```python
from build123d import *

# Parameters (mm, degrees)
F0_R     = 10
F1_DEPTH = 16
F2_R     = 1
F3_R     = 1


with BuildPart() as f1:
    # F0 (on Front) → F1 (new body)
    with BuildSketch(Plane.XZ):
        Polygon((-20, -11.547005), (0, -23.094011), (20, -11.547005), (20, 11.547005), (0, 23.094011), (-20, 11.547005), align=None)
        Circle(F0_R, mode=Mode.SUBTRACT)
    extrude(amount=F1_DEPTH)

    # F2
    f2_edges = [f1.edges().sort_by_distance(p)[0] for p in [
        (-20, -16, 0),
        (-10, -16, -17.320508),
        (10, -16, -17.320508),
        (20, -16, 0),
        (10, -16, 17.320508),
        (-10, -16, 17.320508),
        (-10, -16, 0),
    ]]
    fillet(f2_edges, radius=F2_R)

    # F3
    f3_edges = [f1.edges().sort_by_distance(p)[0] for p in [
        (-20, 0, 0),
        (-10, 0, -17.320508),
        (10, 0, -17.320508),
        (20, 0, 0),
        (10, 0, 17.320508),
        (-10, 0, 17.320508),
        (-10, 0, 0),
    ]]
    fillet(f3_edges, radius=F3_R)


solid = f1.part
```
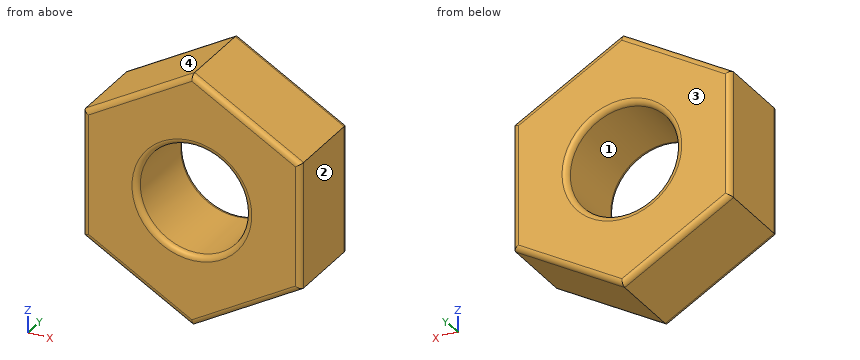
Input: part model. Units: mm. Frame: model coordinates. Face numbers are marked on the shaded views. Give positions to 0.01 mm unless a question says otherwise; leave off trailing zeros. Order: outer loops, then holes, each group sorted by start corner. A loop starts at its lowest first (then second) coordinate and runs counter-clockwise, first axis right, second up. Notation, with made-up numbers: M 50.25,86.5 L 73.25,86.5 A20 cw 73.25,96.5 Z; hole C 70,68.5 d2. An arc over 180 degrees is marked long. One line per question, with ' | ' between items.
1) Ray query, L1, parallel to Y at x = 1, z = 21.5; L2, parallel to Z at x = 3.5, y = -7.25; L3, parallel to X at y = -14.75, z = 8.5. Return the intervals inside material, ascending.
Filled in:
L1: y = -15.99 to -0.01 | L2: z = -21.07 to -9.37, 9.37 to 21.07 | L3: x = -20 to -5.27, 5.27 to 20
2) Draft query along X for the marked faces 1, 2, 3 and 4. Return one class per face: pulls with the +X half, pulls with the -X half, needs draft (parallel to the pull), parting line crosses it, or undercut.
Filled in:
face 1: undercut | face 2: pulls with the +X half | face 3: needs draft | face 4: pulls with the -X half
3) Section A-A on y = -7.75. Output: boundary loops of the cut face in (x, z).
Filled in:
outline: M -20,-11.55 L 0,-23.09 L 20,-11.55 L 20,11.55 L 0,23.09 L -20,11.55 Z; hole C 0,0 d20
4) Section B-B on z = 0. Output: boundary loops of the cut face in (x, y).
Filled in:
outline: M -20,-15 A1 ccw -19,-16 L -11,-16 A1 ccw -10,-15 L -10,-1 A1 ccw -11,0 L -19,0 A1 ccw -20,-1 Z; M 10,-15 A1 ccw 11,-16 L 19,-16 A1 ccw 20,-15 L 20,-1 A1 ccw 19,0 L 11,0 A1 ccw 10,-1 Z
5) Contact query for flat-ended pins moving along their axis: P1, Ø1, axis at y = -3.5, z = 14, coming from the +X side; P2, Ø6, axis at x = -13, y = -2.5, coming from the +Z side; P3, Ø3, axis at x = 3.5, y = -4, coming from the -Z side. Output: stop coordinate, or through.
Filled in:
P1: stops at x = 16.62 | P2: stops at z = 17.32 | P3: stops at z = -21.94
